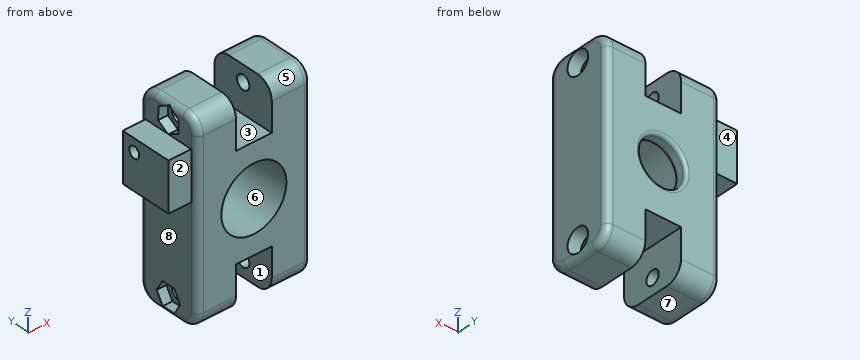
```python
from build123d import *

# Parameters (mm, degrees)
SKETCH1_W           = 35
SKETCH1_H           = 60
BOSS_EXTRUDE1_DEPTH = 20
SKETCH2_R           = 10
CUT_EXTRUDE1_DEPTH  = 16
SKETCH4_R           = 7
CUT_EXTRUDE2_DEPTH  = 42.997755111
FILLET1_R           = 2
SKETCH5_W           = 11
SKETCH5_H           = 14
CUT_EXTRUDE3_DEPTH  = 44.678500826
SKETCH6_R           = 2.15
CUT_EXTRUDE4_DEPTH  = 53.234749007
FILLET3_R           = 5
FILLET4_R           = 5
FILLET7_R           = 1
SKETCH7_W           = 15
SKETCH7_H           = 16
BOSS_EXTRUDE2_DEPTH = 7
SKETCH8_R           = 1.75
CUT_EXTRUDE5_DEPTH  = 15
SKETCH9_R           = 3.6
CUT_EXTRUDE6_DEPTH  = 4
CUT_EXTRUDE7_DEPTH  = 3


with BuildPart() as part:
    # Sketch1 → Boss-Extrude1 (new body)
    with BuildSketch(Plane(origin=(0, 0, 0), x_dir=(1, 0, 0), z_dir=(0, 1, 0))):
        with Locations((-2.608267717, 3.218503937)):
            Rectangle(SKETCH1_W, SKETCH1_H)
    extrude(amount=BOSS_EXTRUDE1_DEPTH)

    # Sketch2 → Cut-Extrude1 (cut)
    with BuildSketch(Plane.XZ):
        with Locations(Location((-2.608267717, -3.218503937, 0), (0, 0, 270))):
            Circle(SKETCH2_R)
    extrude(amount=-CUT_EXTRUDE1_DEPTH, mode=Mode.SUBTRACT)

    # Sketch4 → Cut-Extrude2 (cut, through all)
    with BuildSketch(Plane.XZ.offset(-16)):
        with Locations(Location((-2.608267717, -3.218503937, 0), (0, 0, 270))):
            Circle(SKETCH4_R)
    extrude(amount=-CUT_EXTRUDE2_DEPTH, mode=Mode.SUBTRACT)

    # Fillet1
    fillet1_edges = [part.edges().sort_by_distance(p)[0] for p in [
        (-20.108267717, 20, -3.218503937),
        (14.891732283, 20, -3.218503937),
        (-20.108267717, 0, -3.218503937),
        (14.891732283, 0, -3.218503937),
        (14.891732283, 10, 26.781496063),
        (-20.108267717, 10, 26.781496063),
        (-20.108267717, 10, -33.218503937),
        (14.891732283, 10, -33.218503937),
    ]]
    fillet(fillet1_edges, radius=FILLET1_R)

    # Sketch5 → Cut-Extrude3 (cut, through all)
    with BuildSketch(Plane.XZ):
        with Locations((-2.608267717, 19.781496063)):
            Rectangle(SKETCH5_W, SKETCH5_H)
        with Locations((-2.608267717, -26.218503937)):
            Rectangle(SKETCH5_W, SKETCH5_H)
    extrude(amount=-CUT_EXTRUDE3_DEPTH, mode=Mode.SUBTRACT)

    # Sketch6 → Cut-Extrude4 (cut, through all)
    with BuildSketch(Plane.ZY.offset(20.108267717)):
        with Locations((-28.218503937, 10)):
            Circle(SKETCH6_R)
        with Locations((21.781496063, 10)):
            Circle(SKETCH6_R)
    extrude(amount=-CUT_EXTRUDE4_DEPTH, mode=Mode.SUBTRACT)

    # Fillet3
    # the kernel refuses this fillet: 5 mm, written as the material it takes off along each edge
    with BuildSketch(Plane(origin=(-20.108267717, 15, 21.781496063), x_dir=(0, 0, 1), z_dir=(0, -1, 0))) as fillet3_piece_1:
        with BuildLine():
            CenterArc((3, -2), 2, 0, 90)
            Line((5, -2), (5, 0))
            Line((5, 0), (3, 0))
        make_face()
    revolve(axis=Axis((-20.108267717, 15, 21.781496063), (-1, 0, 0)), revolution_arc=90, mode=Mode.SUBTRACT)
    with BuildSketch(Plane(origin=(-20.108267717, 5, 21.781496063), x_dir=(0, -1, 0), z_dir=(0, 0, -1))) as fillet3_piece_2:
        with BuildLine():
            CenterArc((3, -2), 2, 0, 90)
            Line((5, -2), (5, 0))
            Line((5, 0), (3, 0))
        make_face()
    revolve(axis=Axis((-20.108267717, 5, 21.781496063), (-1, 0, 0)), revolution_arc=90, mode=Mode.SUBTRACT)
    with BuildSketch(Plane(origin=(14.891732283, 15, 21.781496063), x_dir=(0, 1, 0), z_dir=(0, 0, -1))) as fillet3_piece_3:
        with BuildLine():
            CenterArc((3, -2), 2, 0, 90)
            Line((5, -2), (5, 0))
            Line((5, 0), (3, 0))
        make_face()
    revolve(axis=Axis((14.891732283, 15, 21.781496063), (1, 0, 0)), revolution_arc=90, mode=Mode.SUBTRACT)
    with BuildSketch(Plane(origin=(14.891732283, 5, 21.781496063), x_dir=(0, 0, 1), z_dir=(0, 1, 0))) as fillet3_piece_4:
        with BuildLine():
            CenterArc((3, -2), 2, 0, 90)
            Line((5, -2), (5, 0))
            Line((5, 0), (3, 0))
        make_face()
    revolve(axis=Axis((14.891732283, 5, 21.781496063), (1, 0, 0)), revolution_arc=90, mode=Mode.SUBTRACT)
    with BuildSketch(Plane(origin=(4.391732283, 20, 26.781496063), x_dir=(0, 0, -1), z_dir=(-1, 0, 0)), Plane(origin=(14.891732283, 0, 26.781496063), x_dir=(0, 1, 0), z_dir=(-1, 0, 0))) as fillet3_piece_5:
        with BuildLine():
            CenterArc((FILLET3_R, FILLET3_R), FILLET3_R, 180, 90)
            Line((0, FILLET3_R), (0, 0))
            Line((0, 0), (FILLET3_R, 0))
        make_face()
    extrude(amount=24.5, mode=Mode.SUBTRACT)
    with BuildSketch(Plane(origin=(4.391732283, 0, 26.781496063), x_dir=(0, 0, -1), z_dir=(-1, 0, 0)), Plane(origin=(14.891732283, 20, 26.781496063), x_dir=(0, -1, 0), z_dir=(-1, 0, 0))) as fillet3_piece_6:
        with BuildLine():
            CenterArc((FILLET3_R, -FILLET3_R), FILLET3_R, 90, 90)
            Line((0, -FILLET3_R), (0, 0))
            Line((0, 0), (FILLET3_R, 0))
        make_face()
    extrude(amount=24.5, mode=Mode.SUBTRACT)

    # Fillet4
    # the kernel refuses this fillet: 5 mm, written as the material it takes off along each edge
    with BuildSketch(Plane(origin=(-20.108267717, 15, -28.218503937), x_dir=(0, 1, 0), z_dir=(0, 0, 1))) as fillet4_piece_1:
        with BuildLine():
            CenterArc((3, -2), 2, 0, 90)
            Line((5, -2), (5, 0))
            Line((5, 0), (3, 0))
        make_face()
    revolve(axis=Axis((-20.108267717, 15, -28.218503937), (-1, 0, 0)), revolution_arc=90, mode=Mode.SUBTRACT)
    with BuildSketch(Plane(origin=(-20.108267717, 5, -28.218503937), x_dir=(0, 0, -1), z_dir=(0, 1, 0))) as fillet4_piece_2:
        with BuildLine():
            CenterArc((3, -2), 2, 0, 90)
            Line((5, -2), (5, 0))
            Line((5, 0), (3, 0))
        make_face()
    revolve(axis=Axis((-20.108267717, 5, -28.218503937), (-1, 0, 0)), revolution_arc=90, mode=Mode.SUBTRACT)
    with BuildSketch(Plane(origin=(14.891732283, 15, -28.218503937), x_dir=(0, 0, -1), z_dir=(0, -1, 0))) as fillet4_piece_3:
        with BuildLine():
            CenterArc((3, -2), 2, 0, 90)
            Line((5, -2), (5, 0))
            Line((5, 0), (3, 0))
        make_face()
    revolve(axis=Axis((14.891732283, 15, -28.218503937), (1, 0, 0)), revolution_arc=90, mode=Mode.SUBTRACT)
    with BuildSketch(Plane(origin=(14.891732283, 5, -28.218503937), x_dir=(0, -1, 0), z_dir=(0, 0, 1))) as fillet4_piece_4:
        with BuildLine():
            CenterArc((3, -2), 2, 0, 90)
            Line((5, -2), (5, 0))
            Line((5, 0), (3, 0))
        make_face()
    revolve(axis=Axis((14.891732283, 5, -28.218503937), (1, 0, 0)), revolution_arc=90, mode=Mode.SUBTRACT)
    with BuildSketch(Plane(origin=(-9.608267717, 0, -33.218503937), x_dir=(0, 1, 0), z_dir=(1, 0, 0)), Plane(origin=(-20.108267717, 0, -33.218503937), x_dir=(0, 1, 0), z_dir=(1, 0, 0))) as fillet4_piece_5:
        with BuildLine():
            CenterArc((FILLET4_R, FILLET4_R), FILLET4_R, 180, 90)
            Line((0, FILLET4_R), (0, 0))
            Line((0, 0), (FILLET4_R, 0))
        make_face()
    extrude(amount=24.5, mode=Mode.SUBTRACT)
    with BuildSketch(Plane(origin=(-9.608267717, 20, -33.218503937), x_dir=(0, -1, 0), z_dir=(1, 0, 0)), Plane(origin=(-20.108267717, 20, -33.218503937), x_dir=(0, -1, 0), z_dir=(1, 0, 0))) as fillet4_piece_6:
        with BuildLine():
            CenterArc((FILLET4_R, -FILLET4_R), FILLET4_R, 90, 90)
            Line((0, -FILLET4_R), (0, 0))
            Line((0, 0), (FILLET4_R, 0))
        make_face()
    extrude(amount=24.5, mode=Mode.SUBTRACT)

    # Fillet7
    fillet7_edges = [part.edges().sort_by_distance(p)[0] for p in [
        (-2.608267717, 20, 3.781496063),
        (-2.608267717, 16, 3.781496063),
    ]]
    fillet(fillet7_edges, radius=FILLET7_R)

    # Sketch7 → Boss-Extrude2 (add)
    with BuildSketch(Plane.ZY.offset(20.108267717)):
        with Locations((10.281496063, 10)):
            Rectangle(SKETCH7_W, SKETCH7_H)
    extrude(amount=BOSS_EXTRUDE2_DEPTH)

    # Sketch8 → Cut-Extrude5 (cut)
    with BuildSketch(Plane.ZY.offset(27.108267717)):
        with Locations((13.781496063, 14)):
            Circle(SKETCH8_R)
    extrude(amount=-CUT_EXTRUDE5_DEPTH, mode=Mode.SUBTRACT)

    # Sketch9 → Cut-Extrude6 (cut)
    with BuildSketch(Plane(origin=(14.891732283, 0, 0), x_dir=(0, 0, -1), z_dir=(1, 0, 0))):
        with Locations((-21.781496063, 10)):
            Circle(SKETCH9_R)
        with Locations((28.218503937, 10)):
            Circle(SKETCH9_R)
    extrude(amount=-CUT_EXTRUDE6_DEPTH, mode=Mode.SUBTRACT)

    # Sketch10 → Cut-Extrude7 (cut)
    with BuildSketch(Plane.ZY.offset(20.108267717)):
        Polygon((23.74867671, 6.403677763), (25.879592804, 9.905467295), (23.912412157, 13.501789533), (19.814315416, 13.596322237), (17.683399322, 10.094532705), (19.650579969, 6.498210467), align=None)
        Polygon((-24.647931539, 7.986459316), (-24.689440355, 12.085436061), (-28.260012753, 14.098976744), (-31.789076335, 12.013540684), (-31.747567519, 7.914563939), (-28.176995122, 5.901023256), align=None)
    extrude(amount=-CUT_EXTRUDE7_DEPTH, mode=Mode.SUBTRACT)


solid = part.part
```
For this review, take the finished solid that the model builds, in its own axes (mm). Face numbers are marked on the shaded views. A direction names the side the tool comes from. Coordinates: 2 decimals unless noted, no trailing zeros. Order: outer loops, then holes, each group sorted by start corner. A loop starts at its lowest first (then second) coordinate and runs counter-clockwise, first axis right, second up. Notation, with made-up numbers: (82, 71) -> (103, 71) arc R6 cw to (103, 82) -> close; hole circle Ø4 at (71, -39.5). An arc over 180 degrees is marked (long way). Use CSV: the item, a comma, the result in double quotes. Start each with the question number.
Item 1: For the marked faces 1, 2, 3, 4 and 5, list the 3-axis set-ups (+Z, -Z, +X, -X, +Y, -Y) from which the entire face can be reached by the end or side of a thin tool; tool diameter is ignored.
Item 2: Insertion check: pin 1 (5.5 mm diameter, centred on y = 10, z = -28.22, fed in from -X); pin 2 (1.5 mm diameter, centred on y = 4.5, z = -5.5, fed in from -X); pin 3 (3.5 mm diameter, centred on y = 10, z = -28.22, fed in from +X); pin 4 (2 mm diameter, centred on x = -24.5, y = 6.5, fed in from -Z). Each pin has a flat end and moves straight along its axis. Give the tip position at first contact, or say it passes through.
Item 3: Wall thickness on probe 1 along Z at (x, y) = (13, 10); probe 2 along X at (y, z) = (2.75, -22); probe 3 along Z at (x, y) = (13, 7): over which ranges is each line inside the solid? List them lowest first.
Item 4: We need section D-D, the plane y = 11. Give the number of separate pieces and of enclosed holes in the cut face, then the cut area to 3 significant figures.
Item 5: We need section C-C, the plane z = 9. Give the boundary of the cut face in (x, y).
Item 6: Draft analysis for pull direction Z (two halves, no side actions). For the marked faces 6, 7 and 8, state which applies: pulls with the +Z half, pulls with the -Z half, needs draft (parallel to the pull), parting line crosses it, or undercut.
Item 7: We need section B-B, the plane x = -23.5. Give the boundary of the cut face in (y, z), then the cut area to 3 significant figures.
Item 8: We need section A-A, the plane z = -18.5. Give the boundary of the cut face in (x, y).
Derived:
1,face 1,"-Z, +Y, -Y"
1,face 2,"+Z, -Z, -X, -Y"
1,face 3,"+Z, +Y, -Y"
1,face 4,"+Z, -Z, -X, +Y"
1,face 5,"+Z, +X, -X, -Y"
2,pin 1,"stops at x = -17.11"
2,pin 2,"stops at x = -20.11"
2,pin 3,"passes through"
2,pin 4,"stops at z = 2.78"
3,probe 1,"z = -33.22 to -31.82, -24.62 to 18.18, 25.38 to 26.78"
3,probe 2,"x = -20.11 to -8.11, 2.89 to 14.89"
3,probe 3,"z = -33.22 to -30.21, -26.23 to 19.79, 23.77 to 26.78"
4,separate pieces,"5"
4,enclosed holes,"1"
4,area,"1,350 mm^2"
5,outline,"(-27.11, 2) -> (-20.11, 2) arc R2 ccw to (-18.11, 0) -> (12.89, 0) arc R2 ccw to (14.89, 2) -> (14.89, 18) arc R2 ccw to (12.89, 20) -> (-18.11, 20) arc R2 ccw to (-20.11, 18) -> (-27.11, 18) -> close"
6,face 6,"undercut"
6,face 7,"pulls with the -Z half"
6,face 8,"needs draft"
7,outline,"(2, 2.78) -> (18, 2.78) -> (18, 17.78) -> (2, 17.78) -> close; hole circle Ø3.5 at (14, 13.78)"
7,area,"230 mm^2"
8,outline,"(-20.11, 2) arc R2 ccw to (-18.11, 0) -> (12.89, 0) arc R2 ccw to (14.89, 2) -> (14.89, 18) arc R2 ccw to (12.89, 20) -> (-18.11, 20) arc R2 ccw to (-20.11, 18) -> close"
